from build123d import *

# Parameters (mm, degrees)
F0_R     = 12.5
F2_DEPTH = 25
F3_D     = 12
F4_D     = 12


with BuildPart() as f2:
    # F0 (on Front) → F2 (new body, symmetric)
    with BuildSketch(Plane.XZ):
        Circle(F0_R)
    extrude(amount=F2_DEPTH, both=True)

    # F3 (through all)
    with Locations(Plane(origin=(0, 0, 0), x_dir=(0, 1, 0), z_dir=(-1, 0, 0))):
        with Locations((0, 0)):
            Hole(F3_D / 2)

    # F4 (through all)
    with Locations(Plane.YZ):
        with Locations((0, 0)):
            Hole(F4_D / 2)


solid = f2.part
The listing builds one solid part. Answer for the finished solid, in the listing's coordinates (mm). Coordinates: 2 decimals unless noted, no trailing zeros. Write each loop counter-clockwise with the first axis right and the second up, starting at its lowest first coordinate (ties: lowest second). Pieces come first, ordered by that corner, then holes. Notation, with made-up numbers: M 58.5,8 L 78.5,8 A6 cw 78.5,13 Z; hole C 45.25,51.25 d2. An arc over 180 degrees is marked long. Put each result on its own line as item: value. Start each with the question number.
1. A cutting plane is placed at C-C on x = 0. Write down the section's boundary in (y, z).
2. A cutting plane is placed at B-B on x = -7.5. Write down the section's boundary in (y, z), then the cut area to 3 significant figures.
3. Consider line 1 (Z direction, x = -0.5, y = 0); line 2 (Y direction, x = 8, z = -1.5); line 3 (Y direction, x = 9, z = 4). Determine where each line is inside the solid, lowest interval first. Write a range as from..to.
4. A cutting plane is placed at D-D on z = -7.5. Write down the section's boundary in (x, y), then the cut area to 3 significant figures.
5. For a pull along Y with two mould halves and no side action, classify faces 1 (the cylindrical face through (0.171, -5.723, -1.802)), 2 (the flat face through (0, -25, 0)), 3 (the flat face through (0, 25, 0)), 4 (the cylindrical face through (6.72, -0.35, 10.54)) as pulls with the +Y half, pulls with the -Y half, needs draft (parallel to the pull), parting line crosses it, or undercut.
6. Flat-ended cylindrical pins translate along their axes: P1, Ø6, axis at y = 7, z = -4.5, coming from the -X side; P2, Ø2, axis at x = -7, y = -5, coming from the +Z side; P3, Ø8, axis at x = -5.5, y = -10.5, coming from the +Z side. Find the tip coordinate at first contact, or state that the pin passes through.
7. A cutting plane is placed at A-A on z = 0. Write down the section's boundary in (x, y), then the cut area to 3 significant figures.
Resolved:
1. outline: M -25,-12.5 L 25,-12.5 L 25,12.5 L -25,12.5 Z; hole C 0,0 d12
2. outline: M -25,-10 L 25,-10 L 25,10 L -25,10 Z; hole C 0,0 d12
2. area: 887 mm2
3. line 1: z = -12.49..-6, 6..12.49
3. line 2: y = -25..-5.81, 5.81..25
3. line 3: y = -25..-4.47, 4.47..25
4. outline: M -10,-25 L 10,-25 L 10,25 L -10,25 Z
4. area: 1,000 mm2
5. face 1: undercut
5. face 2: pulls with the -Y half
5. face 3: pulls with the +Y half
5. face 4: needs draft
6. P1: stops at x = -12.41
6. P2: stops at z = 10.97
6. P3: stops at z = 12.41
7. outline: M -12.5,-25 L 12.5,-25 L 12.5,-6 L -12.5,-6 Z; M -12.5,6 L 12.5,6 L 12.5,25 L -12.5,25 Z
7. area: 950 mm2
